from build123d import *

# Parameters (mm, degrees)
SKETCH_1_R          = 1.5
SKETCH_1_R_2        = 20
SKETCH_1_R_3        = 5.2
SKETCH_1_R_4        = 2.5
SKETCH_1_W          = 8.4
SKETCH_1_H          = 4.4
EXTRUDE_1_DEPTH     = 4
CUT_EXTRUDE_1_DEPTH = 10


with BuildPart() as part:
    # 草图1 → 凸台-拉伸1 (new body)
    with BuildSketch(Plane.XY):
        with BuildLine():
            Line((-138.972571837, 141.054738201), (21.027428163, 141.054738201))
            Line((21.027428163, 141.054738201), (87.027428163, 75.054738201))
            Line((87.027428163, 75.054738201), (87.027428163, -4.945261799))
            Line((87.027428163, -4.945261799), (16.988248923, -65.708672494))
            ThreePointArc((16.988248923, -65.708672494), (-1.364322077, -66.900830621), (-7.431532599, -49.539175751))
            Line((-7.431532599, -49.539175751), (7.027428163, -4.945261799))
            Line((7.027428163, -4.945261799), (-90.203942848, 92.286109212))
            Line((-90.203942848, 92.286109212), (-138.972571837, 92.286109212))
            Line((-138.972571837, 92.286109212), (-138.972571837, 141.054738201))
        make_face()
        with Locations((-52.972571837, 135.054738201)):
            Circle(SKETCH_1_R, mode=Mode.SUBTRACT)
        with Locations((47.027428163, 15.054738201)):
            Circle(SKETCH_1_R_2, mode=Mode.SUBTRACT)
        with Locations(Location((-22.972571837, 135.054738201, 0), (0, 0, 180))):
            Circle(SKETCH_1_R, mode=Mode.SUBTRACT)
        with Locations((7.027428163, 135.054738201)):
            Circle(SKETCH_1_R, mode=Mode.SUBTRACT)
        with Locations(Location((-112.972571837, 135.054738201, 0), (0, 0, 180))):
            Circle(SKETCH_1_R, mode=Mode.SUBTRACT)
        with Locations((-82.972571837, 135.054738201)):
            Circle(SKETCH_1_R, mode=Mode.SUBTRACT)
        with Locations((7.027428163, -54.227294102)):
            Circle(SKETCH_1_R_3, mode=Mode.SUBTRACT)
        with Locations((49.784787476, 103.812097514)):
            Circle(SKETCH_1_R, mode=Mode.SUBTRACT)
        with Locations(Location((70.997990912, 82.598894078, 0), (0, 0, 180))):
            Circle(SKETCH_1_R, mode=Mode.SUBTRACT)
        with Locations(Location((28.571584041, 125.025300949, 0), (0, 0, 180))):
            Circle(SKETCH_1_R, mode=Mode.SUBTRACT)
        with Locations((-53.337194475, 63.904642213)):
            Circle(SKETCH_1_R, mode=Mode.SUBTRACT)
        with Locations(Location((-32.123991039, 42.691438778, 0), (0, 0, 180))):
            Circle(SKETCH_1_R, mode=Mode.SUBTRACT)
        with Locations(Location((-74.55039791, 85.117845649, 0), (0, 0, 180))):
            Circle(SKETCH_1_R, mode=Mode.SUBTRACT)
        with Locations((70.597428163, 38.624738201)):
            Circle(SKETCH_1_R_4, mode=Mode.SUBTRACT)
        with Locations((70.597428163, -8.515261799)):
            Circle(SKETCH_1_R_4, mode=Mode.SUBTRACT)
        with Locations((23.457428163, -8.515261799)):
            Circle(SKETCH_1_R_4, mode=Mode.SUBTRACT)
        with Locations((23.457428163, 38.624738201)):
            Circle(SKETCH_1_R_4, mode=Mode.SUBTRACT)
        with Locations((-37.972571837, 135.054738201)):
            Rectangle(SKETCH_1_W, SKETCH_1_H, mode=Mode.SUBTRACT)
        with Locations((-7.972571837, 135.054738201)):
            Rectangle(SKETCH_1_W, SKETCH_1_H, mode=Mode.SUBTRACT)
        with Locations((-97.972571837, 135.054738201)):
            Rectangle(SKETCH_1_W, SKETCH_1_H, mode=Mode.SUBTRACT)
        with Locations((-67.972571837, 135.054738201)):
            Rectangle(SKETCH_1_W, SKETCH_1_H, mode=Mode.SUBTRACT)
        Polygon((55.865905794, 94.619709358), (61.805602756, 88.680012396), (64.916872594, 91.791282234), (58.977175632, 97.730979196), align=None, mode=Mode.SUBTRACT)
        Polygon((34.652702359, 115.832912794), (37.763972196, 118.944182631), (43.703669158, 113.004485669), (40.592399321, 109.893215832), align=None, mode=Mode.SUBTRACT)
        Polygon((-47.256076157, 54.712254058), (-41.316379195, 48.772557096), (-38.205109357, 51.883826933), (-44.144806319, 57.823523895), align=None, mode=Mode.SUBTRACT)
        Polygon((-68.469279592, 75.925457494), (-65.358009755, 79.036727331), (-59.418312793, 73.097030369), (-62.52958263, 69.985760532), align=None, mode=Mode.SUBTRACT)
    extrude(amount=EXTRUDE_1_DEPTH)

    # 草图2 → 切除-拉伸1 (cut)
    with BuildSketch(Plane(origin=(0, 0, 0), x_dir=(-1, 0, 0), z_dir=(0, 0, -1))):
        with BuildLine():
            Line((98.792246858, 103.505713788), (110.418981679, 118.616857906))
            ThreePointArc((110.418981679, 118.616857906), (112.113620797, 119.394251765), (113.713072721, 118.436182616))
            Line((113.713072721, 118.436182616), (122.899473042, 103.325038498))
            ThreePointArc((122.899473042, 103.325038498), (122.933741653, 101.305767071), (121.190489151, 100.286109212))
            Line((121.190489151, 100.286109212), (100.377354008, 100.286109212))
            ThreePointArc((100.377354008, 100.286109212), (98.583028348, 101.402709289), (98.792246858, 103.505713788))
        make_face()
        Polygon((127.198237985, 127.054738201), (130.972571837, 120.84615804), (130.972571837, 127.054738201), align=None)
        with BuildLine():
            Line((73.446278945, 98.44171591), (92.214930542, 122.835133626))
            ThreePointArc((92.214930542, 122.835133626), (92.424149051, 124.938138124), (90.629823391, 126.054738201))
            Line((90.629823391, 126.054738201), (32.011635988, 126.054738201))
            ThreePointArc((32.011635988, 126.054738201), (30.086594754, 124.59715524), (30.967460822, 122.348954445))
            Line((30.967460822, 122.348954445), (70.816996628, 97.955536729))
            ThreePointArc((70.816996628, 97.955536729), (72.224826028, 97.694659457), (73.446278945, 98.44171591))
        make_face()
        with BuildLine():
            Line((36.616706696, 93.462689168), (-43.937662379, 92.068564807))
            ThreePointArc((-43.937662379, 92.068564807), (-45.813338133, 93.286939697), (-45.386484011, 95.482478917))
            Line((-45.386484011, 95.482478917), (-23.33185922, 117.537103709))
            Line((-23.33185922, 117.537103709), (-7.607283327, 124.857355573))
            Line((-7.607283327, 124.857355573), (37.626273792, 97.168173472))
            ThreePointArc((37.626273792, 97.168173472), (38.51176098, 94.936649095), (36.616706696, 93.462689168))
        make_face()
        with BuildLine():
            Line((29.20140553, 52.49677533), (-23.612246698, 63.53541151))
            Line((-23.612246698, 63.53541151), (-34.805439363, 70.547080779))
            ThreePointArc((-34.805439363, 70.547080779), (-35.670630649, 72.777688158), (-33.778316178, 74.241693343))
            Line((-33.778316178, 74.241693343), (47.490069377, 75.64817492))
            ThreePointArc((47.490069377, 75.64817492), (49.365745131, 74.42980003), (48.93889101, 72.23426081))
            Line((48.93889101, 72.23426081), (29.20140553, 52.49677533))
        make_face()
    extrude(amount=-CUT_EXTRUDE_1_DEPTH, mode=Mode.SUBTRACT)


solid = part.part
CAD build for the part. Positions are in the model's coordinates, mm. A direction names the side the tool comes from. Give positions to 0.01 mm unless a question says otherwise; leave off trailing zeros. Order: outer loops, then holes, each group sorted by start corner. A loop starts at its lowest first (then second) coordinate and runs counter-clockwise, first axis right, second up. Notation, with made-up numbers: (46, 82) - (58, 82) arc R21 ccw to (58, 113) - close; hole circle Ø5 at (83, 79.25). An arc over 180 degrees is marked (long way). Answer in a Markdown table with one row per item.
1. Flat gauge pin, fed straight in: pin 1 (1.2 mm diameter, centred on x = -37.5, z = 1.5, fed in from -Y). Where does the tip first touch, or does it go through?
Data:
| item | result |
|---|---|
| pin 1 | stops at y = 38.98 |
2. Probe probe 1 along Y at (x, z) = (57, 0.4); probe 2 along Y at (x, z) = (-71, 0.45); probe 3 along X at (y, z) = (114, 3.65). List the from-to ranges inside material, lowest first. Write a range as [from, to].
Data:
| item | result |
|---|---|
| probe 1 | y = [-31, -2.28], [32.39, 93.49], [95.75, 105.08] |
| probe 2 | y = [73.08, 97.86], [126.05, 132.85], [137.25, 141.05] |
| probe 3 | x = [-138.97, -116.41], [-106.87, -85.42], [-44.61, -10.13], [26.87, 36.49], [42.71, 48.08] |
3. Tool access for faces 1 (the flat face through (52.5, -34.9, 2)), 2 (the flat face through (34.51, 106.36, 1.97)): list every direction of +Z, -Z, +X, -X, +Y, -Y with a clear straight run to the whole face (end or side of a thin tool).
Data:
| item | result |
|---|---|
| face 1 | +Z, -Z, +X, -Y |
| face 2 | +Z, -Z |
4. Pull direction X, two halves, no side cores. Call faces 3 (the flat face through (-104.524, 110.956, 1.972)), 4 (the flat face through (53.565, 108.517, 1.972)), 5 (the flat face through (-40.91, 42.99, 1.97)): pulls with the +X half, pulls with the -X half, needs draft (parallel to the pull), parting line crosses it, or undercut.
Data:
| item | result |
|---|---|
| face 3 | undercut |
| face 4 | pulls with the +X half |
| face 5 | pulls with the -X half |
5. Saw through at A-A, the plane z = 1.15. Count the separate pieces of the cut face and the enclosed holes in it, plus the area to 3 significant figures.
Data:
| item | result |
|---|---|
| separate pieces | 1 |
| enclosed holes | 30 |
| area | 18,800 mm² |
6. Saw through at B-B, the plane y = -31.5. Give the cut face in (x, z), plus the area to 3 significant figures.
Data:
| item | result |
|---|---|
| outline | (-1.58, 0) - (56.42, 0) - (56.42, 4) - (-1.58, 4) - close |
| area | 232 mm² |
